Geometry: final body of the model. Coordinates: model frame, mm. Face numbers are marked on the shaded views. A direction names the side the tool comes from. Give positions to 0.01 mm unless a question says otherwise; leave off trailing zeros. Loops run counter-clockwise (first coordinate to the right, second up) from the corner with the lowest first, then second, coordinate; pieces in that order, holes last. Notation, with made-up numbers: (-9.75, -6) -> (8.25, -6) arc R27 ccw to (8.25, 29) -> close; hole circle Ø9 at (-3, 36). An arc over 180 degrees is marked (long way). One line per item, written item: value. Start each with the question number.
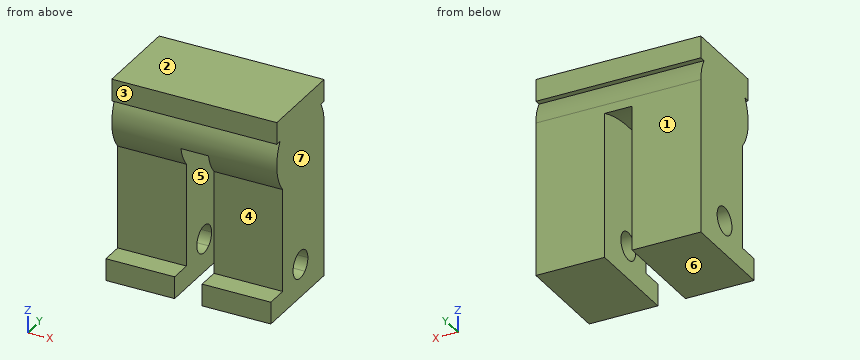
from build123d import *

# Parameters (mm, degrees)
F1_DEPTH = 7.5
F2_R     = 11
F3_DEPTH = 1.25


with BuildPart() as f1:
    # F0 (on Right) → F1 (new body, symmetric)
    with BuildSketch(Plane.YZ):
        with BuildLine():
            Line((4, -1), (4, 1))
            Line((4, 1), (-4, 1))
            Line((-4, 1), (-4, -1))
            Line((-4, -1), (-3.464102, -1))
            ThreePointArc((-3.464102, -1), (-3.980189, -3.397613), (-3, -5.645751))
            Line((-3, -5.645751), (-3, -15))
            Line((-3, -15), (-5, -15))
            Line((-5, -15), (-5, -17))
            Line((-5, -17), (4, -17))
            Line((4, -17), (4, -15))
            Line((4, -15), (4, -3))
            ThreePointArc((4, -3), (3.863703, -1.964724), (3.464102, -1))
            Line((3.464102, -1), (4, -1))
        make_face()
        with BuildLine():
            ThreePointArc((1.25, -14), (1.118034, -14.559017), (0.75, -15))
            ThreePointArc((0.75, -15), (0, -15.25), (-0.75, -15))
            ThreePointArc((-0.75, -15), (-0.559017, -12.881966), (1.25, -14))
        make_face(mode=Mode.SUBTRACT)
    extrude(amount=F1_DEPTH, both=True)

    # F2 (on Right) → F3 (cut, symmetric)
    with BuildSketch(Plane.YZ):
        with Locations((0, -14.027427)):
            Circle(F2_R)
    extrude(amount=F3_DEPTH, both=True, mode=Mode.SUBTRACT)


solid = f1.part
Item 1: Section D-D, the plane y = 2.25. Output: boundary loops of the cut face in (x, z).
Item 2: Mould query, pull axis X, two halves, no side actions, for the marked faces 5, 6 and 7. Classes: pulls with the +X half, pulls with the -X half, needs draft (parallel to the pull), parting line crosses it, or undercut.
Item 3: Section B-B, the plane z = -7.5. Output: boundary loops of the cut face in (x, y), then the cut area to 3 significant figures.
Item 4: Ray query, line 1 along X through (y, z) = (-0.5, -10.25); line 2 along Y through (x, z) = (-2.25, -14); line 3 along Z through (x, y) = (5.25, 0). Return the intervals inside material, ascending. Write a range as [from, to].
Item 5: Section A-A, the plane x = -4.75. Output: boundary loops of the cut face in (y, z).
Item 6: Pin query (flat end, axial travel): pin 1 (2 mm diameter, centred on x = -2.5, z = -7.5, fed in from -Y); pin 2 (1.6 mm diameter, centred on x = 0.5, z = 0, fed in from -Y). Return the tip coordinate at first contact, or that it passes through.
Item 7: Access query for the marked faces 1, 2, 3 and 4. Directions: +Z, -Z, +X, -X, +Y, -Y. A direction counts if a zero-diameter tool reaches every point of the face in a straight line with its end or side. Return the directions, or none.
Item 8: Section C-C, the plane y = 0. Output: boundary loops of the cut face in (x, z), then the cut area to 3 significant figures.
Geometry check:
1. outline: (-7.5, -17) -> (-1.25, -17) -> (-1.25, -3.26) -> (1.25, -3.26) -> (1.25, -17) -> (7.5, -17) -> (7.5, 1) -> (-7.5, 1) -> close
2. face 5: undercut
2. face 6: needs draft
2. face 7: pulls with the +X half
3. outline: (-7.5, -3) -> (-1.25, -3) -> (-1.25, 4) -> (-7.5, 4) -> close; (1.25, -3) -> (7.5, -3) -> (7.5, 4) -> (1.25, 4) -> close
3. area: 87.5 mm2
4. line 1: x = [-7.5, -1.25], [1.25, 7.5]
4. line 2: y = [-3, -1.25], [1.25, 4]
4. line 3: z = [-17, -15.25], [-12.75, 1]
5. outline: (-5, -17) -> (4, -17) -> (4, -3) arc R4 ccw to (3.46, -1) -> (4, -1) -> (4, 1) -> (-4, 1) -> (-4, -1) -> (-3.46, -1) arc R4 ccw to (-3, -5.65) -> (-3, -15) -> (-5, -15) -> close; hole circle Ø2.5 at (0, -14)
6. pin 1: stops at y = -3
6. pin 2: stops at y = -4
7. face 1: +Z, -Z, +X, -X, +Y
7. face 2: +Z, +X, -X, +Y, -Y
7. face 3: +Z, +X, -X, -Y
7. face 4: +X, -X, -Y
8. outline: (-7.5, -17) -> (-1.25, -17) -> (-1.25, -15.25) -> (-7.5, -15.25) -> close; (-7.5, -12.75) -> (-1.25, -12.75) -> (-1.25, -3.03) -> (1.25, -3.03) -> (1.25, -12.75) -> (7.5, -12.75) -> (7.5, 1) -> (-7.5, 1) -> close; (1.25, -17) -> (7.5, -17) -> (7.5, -15.25) -> (1.25, -15.25) -> close
8. area: 204 mm2
